Check sheet for the modelled part. Datum: model origin and axes. Units: mm. Give positions to 0.01 mm unless a question says otherwise; leave off trailing zeros. Order: outer loops, then holes, each group sorted by start corner. A loop starts at its lowest first (then second) coordinate and runs counter-clockwise, first axis right, second up.
```python
from build123d import *

# Parameters (mm, degrees)
BOSS_EXTRUDE2_DEPTH = 5
SKETCH3_R           = 2.75
CUT_EXTRUDE1_DEPTH  = 5


with BuildPart() as part:
    # Sketch1 → Boss-Extrude2 (new body)
    with BuildSketch(Plane(origin=(0, 0, 0), x_dir=(1, 0, 0), z_dir=(0, 1, 0))):
        with BuildLine():
            Line((10, 0), (160, 0))
            ThreePointArc((160, 0), (167.071067812, 2.928932188), (170, 10))
            Line((170, 10), (170, 50))
            ThreePointArc((170, 50), (167.071067812, 57.071067812), (160, 60))
            Line((160, 60), (10, 60))
            ThreePointArc((10, 60), (2.928932188, 57.071067812), (0, 50))
            Line((0, 50), (0, 10))
            ThreePointArc((0, 10), (2.928932188, 2.928932188), (10, 0))
        make_face()
    extrude(amount=BOSS_EXTRUDE2_DEPTH)

    # Sketch3 → Cut-Extrude1 (cut)
    with BuildSketch(Plane(origin=(0, 5, 0), x_dir=(1, 0, 0), z_dir=(0, 1, 0))):
        with Locations(Location((5, 30, 0), (0, 0, 270))):
            Circle(SKETCH3_R)
        with Locations(Location((45, 55, 0), (0, 0, 270))):
            Circle(SKETCH3_R)
        with Locations(Location((125, 55, 0), (0, 0, 270))):
            Circle(SKETCH3_R)
        with Locations(Location((165, 30, 0), (0, 0, 270))):
            Circle(SKETCH3_R)
        with Locations(Location((125, 5, 0), (0, 0, 270))):
            Circle(SKETCH3_R)
        with Locations(Location((45, 5, 0), (0, 0, 270))):
            Circle(SKETCH3_R)
    extrude(amount=-CUT_EXTRUDE1_DEPTH, mode=Mode.SUBTRACT)


solid = part.part
```
(1) Gauge pin test, flat end, axial feed: pin 1 Ø5 at (x, z) = (45, -55) entering from -Y. Record the tip position at first contact, or that the pin passes through.
Response values:
pin 1: passes through
(2) Material ranges on L1, parallel to X at y = 1.3, z = -30; L2, parallel to X at y = 3.1, z = -53; L3, parallel to Z at x = 165, y = 1.2, recorded low to high.
Response values:
L1: x = 0 to 2.25, 7.75 to 162.25, 167.75 to 170
L2: x = 0.46 to 43.11, 46.89 to 123.11, 126.89 to 169.54
L3: z = -58.66 to -32.75, -27.25 to -1.34
(3) Cross-section at A-A on x = 45. Enter the section's corners in (y, z).
Response values:
outline: (0, -60) - (5, -60) - (5, -57.75) - (0, -57.75) - close; (0, -52.25) - (5, -52.25) - (5, -7.75) - (0, -7.75) - close; (0, -2.25) - (5, -2.25) - (5, 0) - (0, 0) - close
(4) Release check for a two-part mould opening along X. For faces 1 (the face through (0, 2, -30)), 2 (the face through (84, 0, -30)), 3 (the face through (123.327, 2.535, -57.182)) record: released by +X, released by -X, zero draft, split by the parting line, or undercut.
Response values:
face 1: released by -X
face 2: zero draft
face 3: undercut
(5) Cross-section at C-C on z = -31. Enter the section's corners in (x, y), then the cut area to 3 significant figures.
Response values:
outline: (0, 0) - (2.44, 0) - (2.44, 5) - (0, 5) - close; (7.56, 0) - (162.44, 0) - (162.44, 5) - (7.56, 5) - close; (167.56, 0) - (170, 0) - (170, 5) - (167.56, 5) - close
area: 799 mm2
(6) Cross-section at B-B on y = 3.2. Enter the section's corners in (x, z).
Response values:
outline: (0, -50) arc R10 ccw to (10, -60) - (160, -60) arc R10 ccw to (170, -50) - (170, -10) arc R10 ccw to (160, 0) - (10, 0) arc R10 ccw to (0, -10) - close; hole circle Ø5.5 at (5, -30); hole circle Ø5.5 at (45, -55); hole circle Ø5.5 at (45, -5); hole circle Ø5.5 at (125, -55); hole circle Ø5.5 at (125, -5); hole circle Ø5.5 at (165, -30)
(7) Cross-section at D-D on x = 165. Enter the section's corners in (y, z).
Response values:
outline: (0, -58.66) - (5, -58.66) - (5, -32.75) - (0, -32.75) - close; (0, -27.25) - (5, -27.25) - (5, -1.34) - (0, -1.34) - close
